from build123d import *

# Parameters (mm, degrees)
F0_W     = 5
F0_H     = 5
F1_DEPTH = 10


with BuildPart() as f1:
    # F0 (on Top) → F1 (new body)
    with BuildSketch(Plane.XY):
        Polygon((-10, 10), (-115, 10), (-115, -10), (-10, -10), (-10, -5), (-105, -5), (-105, 5), (-10, 5), align=None)
        Polygon((-10, 75), (-10, 10), (-5, 10), (-5, 65), (5, 65), (5, 10), (10, 10), (10, 75), align=None)
        with Locations((-7.5, 7.5)):
            Rectangle(F0_W, F0_H)
        with Locations((-7.5, -7.5)):
            Rectangle(F0_W, F0_H)
        Polygon((-5, -10), (-10, -10), (-10, -75), (10, -75), (10, -10), (5, -10), (5, -65), (-5, -65), align=None)
        with Locations((7.5, 7.5)):
            Rectangle(F0_W, F0_H)
        Polygon((115, 10), (10, 10), (10, 5), (105, 5), (105, -5), (10, -5), (10, -10), (115, -10), align=None)
        with Locations((7.5, -7.5)):
            Rectangle(F0_W, F0_H)
    extrude(amount=F1_DEPTH)


solid = f1.part
For this review, take the finished solid that the model builds, in its own axes (mm). A direction names the side the tool comes from. Coordinates: 2 decimals unless noted, no trailing zeros. Loops run counter-clockwise (first coordinate to the right, second up) from the corner with the lowest first, then second, coordinate; pieces in that order, holes last. Notation, with made-up numbers: (68, 39.25) - (116, 39.25) arc R5 ccw to (116, 43.25) - close; hole circle Ø4 at (58, 53.25). An arc over 180 degrees is marked (long way). Return JSON: item names as keys, results as strings.
Item 1: For line 1 (X direction, y = -43, z = 1.25); line 2 (Y direction, x = 3, z = 4.5), list the stretches that pass through material, from the lowest coordinate up.
Determined:
{"line 1": "x = -10 to -5, 5 to 10", "line 2": "y = -75 to -65, 65 to 75"}
Item 2: For faces 5 (the flat face through (10, 42, 5)), 6 (the flat face through (-10, 43, 5)), 7 (the flat face through (5, -35, 5)), 8 (the flat face through (-10, -42, 5)), 9 (the flat face through (-115, 0, 5)), list the 3-axis set-ups (+Z, -Z, +X, -X, +Y, -Y) from which the entire face can be reached by the end or side of a thin tool; tool diameter is ignored.
Determined:
{"face 5": "+Z, -Z, +X, +Y", "face 6": "+Z, -Z, -X, +Y", "face 7": "+Z, -Z", "face 8": "+Z, -Z, -X, -Y", "face 9": "+Z, -Z, -X, +Y, -Y"}
Item 3: Take a section at C-C (z = 4). Give the boundary of the cut face in (x, y).
Determined:
{"outline": "(-115, -10) - (-10, -10) - (-10, -75) - (10, -75) - (10, -10) - (115, -10) - (115, 10) - (10, 10) - (10, 75) - (-10, 75) - (-10, 10) - (-115, 10) - close; hole (-105, -5) - (-5, -5) - (-5, -65) - (5, -65) - (5, -5) - (105, -5) - (105, 5) - (5, 5) - (5, 65) - (-5, 65) - (-5, 5) - (-105, 5) - close"}
Item 4: Insertion check: pin 1 (6 mm diameter, centred on x = -81, z = 7.5, fed in from -Y); pin 2 (5 mm diameter, centred on y = -20.5, z = 8, fed in from +X); pin 3 (1.5 mm diameter, centred on x = -69.5, z = 2, fed in from +Y). Each pin has a flat end and moves straight along its axis. Give the tip position at first contact, or say it passes through.
Determined:
{"pin 1": "stops at y = -10", "pin 2": "stops at x = 10", "pin 3": "stops at y = 10"}
Item 5: Mouldability with a two-part tool opening along Y and no side actions: class faces 1 (the flat face through (10, -43, 5)), 2 (the flat face through (63, 10, 5)), 3 (the flat face through (-5, 35, 5)), 4 (the flat face through (62, -10, 5)) as pulls with the +Y half, pulls with the -Y half, needs draft (parallel to the pull), parting line crosses it, or undercut.
Determined:
{"face 1": "needs draft", "face 2": "pulls with the +Y half", "face 3": "undercut", "face 4": "pulls with the -Y half"}
Item 6: Take a section at A-A (y = -19.5). Give the boundary of the cut face in (x, z), then the cut area to 3 significant figures.
Determined:
{"outline": "(-10, 0) - (-5, 0) - (-5, 10) - (-10, 10) - close; (5, 0) - (10, 0) - (10, 10) - (5, 10) - close", "area": "100 mm2"}
